from build123d import *

# Parameters (mm, degrees)
BOSS_EXTRUDE1_DEPTH = 2
SKETCH2_OUTSIDE_W   = 24.844
SKETCH2_OUTSIDE_H   = 23.504
SKETCH2_OUTSIDE_R   = 4.330127019
CUT_EXTRUDE2_DEPTH  = 8.729812417
CUT_EXTRUDE2_DRAFT  = -30
SKETCH3_R           = 2.5
BOSS_EXTRUDE2_DEPTH = 9


with BuildPart() as part:
    # Sketch1 → Boss-Extrude1 (new, symmetric)
    with BuildSketch(Plane(origin=(0, 0, 0), x_dir=(1, 0, 0), z_dir=(0, 1, 0))):
        Polygon((5, 0), (2.5, 4.330127019), (-2.5, 4.330127019), (-5, 0), (-2.5, -4.330127019), (2.5, -4.330127019), align=None)
    extrude(amount=BOSS_EXTRUDE1_DEPTH, both=True)


with BuildPart() as cut_extrude2_tool:
    # Sketch2 outside → Cut-Extrude2 (with draft: the straight prism first)
    with BuildSketch(Plane(origin=(0, 2, 0), x_dir=(1, 0, 0), z_dir=(0, 1, 0))):
        Rectangle(SKETCH2_OUTSIDE_W, SKETCH2_OUTSIDE_H)
        Circle(SKETCH2_OUTSIDE_R, mode=Mode.SUBTRACT)
    extrude(amount=-CUT_EXTRUDE2_DEPTH)
    # Cut-Extrude2: the draft: its side faces are tilted about the plane it starts from
    cut_extrude2_sides = [cut_extrude2_tool.faces().sort_by_distance(p)[0] for p in [
        (0, -2.364906208, 11.752),
        (12.422, -2.364906208, 0),
        (0, -2.364906208, -11.752),
        (-12.422, -2.364906208, 0),
        (-4.330127019, -2.364906208, 0),
    ]]
    draft(cut_extrude2_sides, Plane(origin=(0, 2, 0), x_dir=(1, 0, 0), z_dir=(0, 1, 0)), CUT_EXTRUDE2_DRAFT)


with BuildPart() as part_1:
    add(part.part)

    # Cut-Extrude2: cut by cut_extrude2_tool
    add(cut_extrude2_tool.part, mode=Mode.SUBTRACT)

    # Sketch3 → Boss-Extrude2 (add)
    with BuildSketch(Plane.XZ.offset(2)):
        with Locations(Location((0, 0, 0), (0, 0, 270))):
            Circle(SKETCH3_R)
    extrude(amount=BOSS_EXTRUDE2_DEPTH)


solid = part_1.part
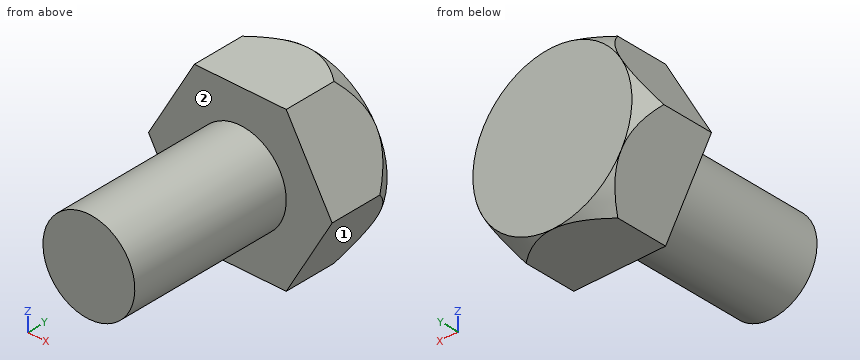
Model file for the job. Use its own axes, mm. Face numbers are marked on the shaded views. A direction names the side the tool comes from. Give positions to 0.01 mm unless a question says otherwise; leave off trailing zeros. Order: outer loops, then holes, each group sorted by start corner. A loop starts at its lowest first (then second) coordinate and runs counter-clockwise, first axis right, second up. Notation, with made-up numbers: M -26,31 L 22,31 A4 ccw 22,36 Z; hole C -21,51 d6. An arc over 180 degrees is marked long. Put each result on its own line as item: value. Start each with the question number.
(1) Drill centre lines: L1, parallel to Y at x = -2.75, z = -1; L2, parallel to Z at x = 3.75, y = 0.5. Where is each one in solid material? Low to high. Write a range as [from, to].
(2) Pin check, flat tips, straight feed: pin 1 Ø4 at (y, z) = (-6, 2.5) entering from -X; pin 2 Ø4 at (x, y) = (-3, -5) entering from +Z. Stop position of each tip, or through.
(3) Tool access for the marked faces 1 and 2: list every direction of +Z, -Z, +X, -X, +Y, -Y with a clear straight run to the whole face (end or side of a thin tool).
(4) Band-saw the part on A-A on y = -6.75. Give the cut face in (x, z).
Results below:
1. L1: y = [-2, 2]
1. L2: z = [-2.17, 2.17]
2. pin 1: stops at x = -2.45
2. pin 2: stops at z = 2.29
3. face 1: -Z, +X, +Y, -Y
3. face 2: -Y
4. outline: C 0,0 d5
